The model under review builds one solid part; all positions refer to its coordinate system, in mm. A direction names the side the tool comes from. Coordinates: 2 decimals unless noted, no trailing zeros. Write each loop counter-clockwise with the first axis right and the second up, starting at its lowest first coordinate (ties: lowest second). Pieces come first, ordered by that corner, then holes. Notation, with made-up numbers: (36.5, 31) - (63.5, 31) arc R35 ccw to (63.5, 69) - close; hole circle Ø10 at (50.5, 20). An arc over 180 degrees is marked (long way). Return JSON: item names as keys, results as strings. Group by question number.
(1) Tool access review of faces 1 (the face through (33, 1, 31)), 2 (the face through (0, 1, 34)), 3 (the face through (-1, 2, 0)): name each direction out of +Z, -Z, +X, -X, +Y, -Y from which nothing blocks a thin tool from reaching the whole face with its end or side.
(2) For pin 1 Ø0.9 at (y, z) = (2, -23.5) entering from -X; pin 2 Ø1 at (y, z) = (2, -24.5) entering from +X; pin 3 Ø0.9 at (y, z) = (2, -31.5) entering from +X, all flat-tipped, find the tip position at first contact; note any pin that passes through.
(3) We need section B-B on x = -37. State the section outline as (y, z) points, then the cut area to 3 significant figures.
(4) Draft analysis for pull direction X (two halves, no side actions). For faces 4 (the face through (36.169, 1.479, 16.596)), 5 (the face through (42.7, 1.5, -24.2)), 6 (the face through (-33, 1, 24)), state which applies: released by +X, released by -X, zero draft, split by the parting line, or undercut.
(5) We need section D-D on x = 10.5. State the section outline as (y, z) points.
(6) We need section C-C on y = 2.5. State the section outline as (x, z) points.
(7) To check wall thickness, follow L1, parallel to Z at x = 7.5, y = 2.05; L2, parallel to X at y = 2.4, z = 3.5; L3, parallel to Y at x = 3, z = -12.5. State the ranges of each line that lie inside material, in increasing order. Write a range as from..to.
(8) We need section A-A on z = 0. State the section outline as (x, y) points.
```python
from build123d import *

# Parameters (mm, degrees)
SKETCH1_R           = 1.8
BOSS_EXTRUDE1_DEPTH = 3
CUT_EXTRUDE1_START  = 3
SKETCH3_W           = 57.25
SKETCH3_H           = 62.7
CUT_EXTRUDE1_DEPTH  = 1


with BuildPart() as part:
    # Sketch1 → Boss-Extrude1 (new body)
    with BuildSketch(Plane(origin=(0, 0, 0), x_dir=(-1, 0, 0), z_dir=(0, 1, 0))):
        with BuildLine():
            Line((-33, 29.381966011), (-33, 33))
            ThreePointArc((-33, 33), (-32.707106781, 33.707106781), (-32, 34))
            Line((-32, 34), (32, 34))
            ThreePointArc((32, 34), (32.707106781, 33.707106781), (33, 33))
            Line((33, 33), (33, 14.381966011))
            Line((33, 14.381966011), (41.894427191, 9.934752416))
            ThreePointArc((41.894427191, 9.934752416), (42.701301617, 9.197360258), (43, 8.145898034))
            Line((43, 8.145898034), (43, -8.145898034))
            ThreePointArc((43, -8.145898034), (42.701301617, -9.197360258), (41.894427191, -9.934752416))
            Line((41.894427191, -9.934752416), (33, -14.381966011))
            Line((33, -14.381966011), (33, -33))
            ThreePointArc((33, -33), (32.707106781, -33.707106781), (32, -34))
            Line((32, -34), (-32, -34))
            ThreePointArc((-32, -34), (-32.707106781, -33.707106781), (-33, -33))
            Line((-33, -33), (-33, -29.381966011))
            Line((-33, -29.381966011), (-41.894427191, -24.934752416))
            ThreePointArc((-41.894427191, -24.934752416), (-42.701301617, -24.197360258), (-43, -23.145898034))
            Line((-43, -23.145898034), (-43, 23.145898034))
            ThreePointArc((-43, 23.145898034), (-42.701301617, 24.197360258), (-41.894427191, 24.934752416))
            Line((-41.894427191, 24.934752416), (-33, 29.381966011))
        make_face()
        with Locations((-37, 18.192906379)):
            Circle(SKETCH1_R, mode=Mode.SUBTRACT)
        with Locations((-37, -18.896413475)):
            Circle(SKETCH1_R, mode=Mode.SUBTRACT)
        with Locations((37, 0)):
            Circle(SKETCH1_R, mode=Mode.SUBTRACT)
    extrude(amount=BOSS_EXTRUDE1_DEPTH)

    # Sketch3 → Cut-Extrude1 (cut)
    with BuildSketch(Plane(origin=(0, 0, 0), x_dir=(-1, 0, 0), z_dir=(0, 1, 0)).offset(CUT_EXTRUDE1_START)):
        with Locations((1.775, 0)):
            Rectangle(SKETCH3_W, SKETCH3_H)
    extrude(amount=-CUT_EXTRUDE1_DEPTH, mode=Mode.SUBTRACT)


solid = part.part
```
Ans:
{
 "1": {"face 1": "+Z, +X, +Y, -Y", "face 2": "+Z, +X, -X, +Y, -Y", "face 3": "+Y"},
 "2": {"pin 1": "x = -33", "pin 2": "x = 42.81", "pin 3": "x = 33"},
 "3": {"outline": "(0, -12.38) - (3, -12.38) - (3, -1.8) - (0, -1.8) - close; (0, 1.8) - (3, 1.8) - (3, 12.38) - (0, 12.38) - close", "area": "63.5 mm²"},
 "4": {"face 4": "undercut", "face 5": "released by +X", "face 6": "released by -X"},
 "5": {"outline": "(0, -34) - (3, -34) - (3, -31.35) - (2, -31.35) - (2, 31.35) - (3, 31.35) - (3, 34) - (0, 34) - close"},
 "6": {"outline": "(-43, -8.15) arc R2 ccw to (-41.89, -9.93) - (-33, -14.38) - (-33, -33) arc R1 ccw to (-32, -34) - (32, -34) arc R1 ccw to (33, -33) - (33, -29.38) - (41.89, -24.93) arc R2 ccw to (43, -23.15) - (43, 23.15) arc R2 ccw to (41.89, 24.93) - (33, 29.38) - (33, 33) arc R1 ccw to (32, 34) - (-32, 34) arc R1 ccw to (-33, 33) - (-33, 14.38) - (-41.89, 9.93) arc R2 ccw to (-43, 8.15) - close; hole circle Ø3.6 at (-37, 0); hole (-30.4, -31.35) - (26.85, -31.35) - (26.85, 31.35) - (-30.4, 31.35) - close; hole circle Ø3.6 at (37, -18.9); hole circle Ø3.6 at (37, 18.19)"},
 "7": {"L1": "-34..-31.35, 31.35..34", "L2": "-43..-30.4, 26.85..43", "L3": "0..2"},
 "8": {"outline": "(-43, 0) - (-38.8, 0) - (-38.8, 3) - (-43, 3) - close; (-35.2, 0) - (43, 0) - (43, 3) - (26.85, 3) - (26.85, 2) - (-30.4, 2) - (-30.4, 3) - (-35.2, 3) - close"}
}
